from build123d import *

# Parameters (mm, degrees)
SKETCH_1_R               = 26
EXTRUDE_1_DEPTH          = 4
SKETCH_2_R               = 18
EXTRUDE_2_DEPTH          = 19.3
SKETCH_3_R               = 13
CUT_EXTRUDE_1_DEPTH      = 10.3
SKETCH_6_R               = 13
CUT_EXTRUDE_4_DEPTH      = 14
SKETCH_7_R               = 1
CUT_EXTRUDE_5_DEPTH      = 5
SKETCH_8_R               = 28
SKETCH_8_R_2             = 26
EXTRUDE_3_DEPTH          = 6
CHAMFER_1_SIZE           = 0.5
CHAMFER_2_SIZE           = 0.5
PATTERN_CIRCULAR_1_COUNT = 4
SKETCH_10_R              = 15
CUT_EXTRUDE_7_DEPTH      = 11.8
SKETCH_11_R              = 15
SKETCH_11_R_2            = 12
EXTRUDE_4_DEPTH          = 2
SKETCH_12_R              = 2
CUT_EXTRUDE_8_DEPTH      = 10


with BuildPart() as part:
    # Эскиз1 → Бобышка-Вытянуть1 (new body)
    with BuildSketch(Plane(origin=(0, 0, 0), x_dir=(1, 0, 0), z_dir=(0, 1, 0))):
        Circle(SKETCH_1_R)
    extrude(amount=EXTRUDE_1_DEPTH)

    # Эскиз2 → Бобышка-Вытянуть2 (add)
    with BuildSketch(Plane(origin=(0, 4, 0), x_dir=(1, 0, 0), z_dir=(0, 1, 0))):
        Circle(SKETCH_2_R)
    extrude(amount=EXTRUDE_2_DEPTH)

    # Эскиз3 → Вырез-Вытянуть1 (cut)
    with BuildSketch(Plane(origin=(0, 23.3, 0), x_dir=(1, 0, 0), z_dir=(0, 1, 0))):
        Circle(SKETCH_3_R)
    extrude(amount=-CUT_EXTRUDE_1_DEPTH, mode=Mode.SUBTRACT)

    # Эскиз6 → Вырез-Вытянуть4 (cut, through all)
    with BuildSketch(Plane(origin=(0, 13, 0), x_dir=(1, 0, 0), z_dir=(0, 1, 0))):
        Circle(SKETCH_6_R)
    extrude(amount=-CUT_EXTRUDE_4_DEPTH, mode=Mode.SUBTRACT)

    # Эскиз7 → Вырез-Вытянуть5 (cut)
    with BuildSketch(Plane(origin=(0, 23.3, 0), x_dir=(1, 0, 0), z_dir=(0, 1, 0))):
        with Locations((-15.5, 0)):
            Circle(SKETCH_7_R)
        with Locations((0, 15.5)):
            Circle(SKETCH_7_R)
        with Locations((15.5, 0)):
            Circle(SKETCH_7_R)
        with Locations((0, -15.5)):
            Circle(SKETCH_7_R)
    extrude(amount=-CUT_EXTRUDE_5_DEPTH, mode=Mode.SUBTRACT)

    # Эскиз8 → Бобышка-Вытянуть3 (add)
    with BuildSketch(Plane(origin=(0, 4, 0), x_dir=(1, 0, 0), z_dir=(0, 1, 0))):
        Circle(SKETCH_8_R)
        Circle(SKETCH_8_R_2, mode=Mode.SUBTRACT)
    extrude(amount=-EXTRUDE_3_DEPTH)

    # Фаска1
    chamfer_1_edges = [part.edges().sort_by_distance(p)[0] for p in [
        (-26, -2, 0),
    ]]
    chamfer(chamfer_1_edges, length=CHAMFER_1_SIZE)

    # Фаска2
    chamfer_2_edges = [part.edges().sort_by_distance(p)[0] for p in [
        (-18, 23.3, 0),
    ]]
    chamfer(chamfer_2_edges, length=CHAMFER_2_SIZE)

    # Эскиз9 → Вырез-Повернуть2 (revolve, cut)
    with BuildSketch(Plane(origin=(0, 0, 0), x_dir=(0, 0, -1), z_dir=(1, 0, 0))):
        Polygon((-20.9, 2.648035715), (-19.5, 4), (-22, 4), (-22, 2.648035715), (-22, -2), (-20.9, -2), align=None)
    cut_revolve_2 = revolve(axis=Axis((0, -20.768821294, 22), (0, 1, 0)), mode=Mode.SUBTRACT)

    # Круговой массив1: Вырез-Повернуть2 ×4 about axis
    pattern_circular_1_axis = Axis((0, 0, 0), (0, 1, 0))
    for i in range(1, PATTERN_CIRCULAR_1_COUNT):
        add(cut_revolve_2.rotate(pattern_circular_1_axis, i * 360 / PATTERN_CIRCULAR_1_COUNT), mode=Mode.SUBTRACT)

    # Эскиз10 → Вырез-Вытянуть7 (cut)
    with BuildSketch(Plane.XZ):
        Circle(SKETCH_10_R)
    extrude(amount=-CUT_EXTRUDE_7_DEPTH, mode=Mode.SUBTRACT)

    # Эскиз11 → Бобышка-Вытянуть4 (add)
    with BuildSketch(Plane.XZ.offset(-11.8)):
        Circle(SKETCH_11_R)
        Circle(SKETCH_11_R_2, mode=Mode.SUBTRACT)
    extrude(amount=EXTRUDE_4_DEPTH)

    # Эскиз12 → Вырез-Вытянуть8 (cut)
    with BuildSketch(Plane(origin=(0, 4, 0), x_dir=(1, 0, 0), z_dir=(0, 1, 0))):
        with Locations((15.556349186, -15.556349186)):
            Circle(SKETCH_12_R)
    extrude(amount=-CUT_EXTRUDE_8_DEPTH, mode=Mode.SUBTRACT)


solid = part.part
Verification items for the finished model (mm, model axes). A direction names the side the tool comes from. Give positions to 0.01 mm unless a question says otherwise; leave off trailing zeros. Write each loop counter-clockwise with the first axis right and the second up, starting at its lowest first coordinate (ties: lowest second). Pieces come first, ordered by that corner, then holes. Notation, with made-up numbers: M -39,33 L -29,33 A21 ccw -29,72 Z; hole C -29,-16.75 d6. An arc over 180 degrees is marked long. Write item = value, one per line.
(1) Access from +Z, -Z, +X, -X, +Y, -Y to the whole of each face (thin tool, end or side, straight path). Record for faces 1 (the face through (23.1, 1.3, 0)), 2 (the face through (-7, 9.8, 10)), 3 (the face through (-0.217, 20.835, -14.524)).
Found:
face_1 = +Y, -Y
face_2 = -Y
face_3 = +Y
(2) Go/stop test with flat-tipped pins: pin 1 Ø3 at (x, z) = (0, -15.5) entering from +Y; pin 2 Ø4 at (x, y) = (-3.5, 16) entering from +Z; pin 3 Ø2 at (x, z) = (-17.5, 18.5) entering from -Y; pin 4 Ø3.5 at (x, z) = (0, 22) entering from +Y. Record where each tip stops, or that it passes through.
Found:
pin_1 = 23.3
pin_2 = 17.94
pin_3 = -1.97
pin_4 = 3.28
(3) Sectioned sample at B-B (y = 8.75). Record the cut outline in (x, z), then the cut area to 3 significant figures.
Found:
outline = C 0,0 d36; hole C 0,0 d30
area = 311 mm2
(4) Sectioned sample at A-A (x = 0). Give the number of separate pieces and of enclosed holes in the cut face, then the cut area to 3 significant figures.
Found:
separate_pieces = 4
enclosed_holes = 0
area = 244 mm2
(5) Material ranges on line 1 (Z direction, x = 0, y = -0.8); line 2 (X direction, y = 3, z = -9); line 3 (Y direction, x = 20, z = 16), recorded low to high.
Found:
line_1 = -28 to -26, 26 to 28
line_2 = -26.51 to -12, 12 to 26.51
line_3 = 0 to 4
